Here's how the part is built. I have some questions about the finished solid (model axes, mm). Round coordinates to 2 decimals unless told otherwise and drop trailing zeros. Write each loop counter-clockwise with the first axis right and the second up, starting at its lowest first coordinate (ties: lowest second). Pieces come first, ordered by that corner, then holes. Notation, with made-up numbers: (-13, -12) -> (19, -12) arc R23 ccw to (19, 17) -> close; hole circle Ø2 at (-15.75, 36). An arc over 180 degrees is marked (long way). Answer in a Markdown table with one row per item.
from build123d import *

# Parameters (mm, degrees)
F0_R     = 15.875
F1_DEPTH = 25.4


with BuildPart() as f1:
    # F0 (on Front) → F1 (new body)
    with BuildSketch(Plane.XZ):
        with BuildLine():
            ThreePointArc((-49.0055754781, -12.3038528651), (-41.5660877202, -30.2643651072), (-23.6055754781, -37.7038528651))
            Line((-23.6055754781, -37.7038528651), (-23.3435511934, -37.7038528651))
            Line((-23.3435511934, -37.7038528651), (42.6555754781, -37.7038528651))
            ThreePointArc((42.6555754781, -37.7038528651), (60.6160877202, -30.2643651072), (68.0555754781, -12.3038528651))
            ThreePointArc((68.0555754781, -12.3038528651), (66.5394936483, -3.6598692442), (62.1722327349, 3.9522256755))
            Line((62.1722327349, 3.9522256755), (31.7932017285, 51.9582280247))
            Line((31.7932017285, 51.9582280247), (30.1001638771, 54.6336253754))
            ThreePointArc((30.1001638771, 54.6336253754), (9.0757549966, 65.1359410719), (-11.5640531978, 53.8966029481))
            Line((-11.5640531978, 53.8966029481), (-12.2938214906, 52.7437224792))
            Line((-12.2938214906, 52.7437224792), (-43.3631999383, 3.6606368673))
            ThreePointArc((-43.3631999383, 3.6606368673), (-47.5104832797, -3.714089206), (-49.0055754781, -12.0418285804))
            Line((-49.0055754781, -12.0418285804), (-49.0055754781, -12.3038528651))
        make_face()
        with Locations((-23.6055754781, -12.3038528651)):
            Circle(F0_R, mode=Mode.SUBTRACT)
        with BuildLine():
            ThreePointArc((26.7805754781, -12.3038528651), (42.6555754781, 3.5711471349), (58.5305754781, -12.3038528651))
            ThreePointArc((58.5305754781, -12.3038528651), (42.6555754781, -28.1788528651), (26.7805754781, -12.3038528651))
        make_face(mode=Mode.SUBTRACT)
        with Locations((9.525, 39.7399142385)):
            Circle(F0_R, mode=Mode.SUBTRACT)
        with BuildLine():
            Line((-23.3435511934, -37.7038528651), (-23.6055754781, -37.7038528651))
            ThreePointArc((-23.6055754781, -37.7038528651), (-41.5660877202, -30.2643651072), (-49.0055754781, -12.3038528651))
            Line((-49.0055754781, -12.3038528651), (-49.0055754781, -12.0418285804))
            ThreePointArc((-49.0055754781, -12.0418285804), (-41.5670433569, -30.2653207439), (-23.3435511934, -37.7038528651))
        make_face()
        with BuildLine():
            ThreePointArc((-11.5640531978, 53.8966029481), (-11.936680058, 53.3250638176), (-12.2938214906, 52.7437224792))
            Line((-12.2938214906, 52.7437224792), (-11.5640531978, 53.8966029481))
        make_face()
        with BuildLine():
            Line((30.1001638771, 54.6336253754), (31.7932017285, 51.9582280247))
            ThreePointArc((31.7932017285, 51.9582280247), (30.9884091386, 53.3223318491), (30.1001638771, 54.6336253754))
        make_face()
    extrude(amount=F1_DEPTH)


solid = f1.part
1) I want a section at B-B, the plane x = 15. List the corners of the cut face in (y, z) for me.
Response:
| item | result |
|---|---|
| outline | (-25.4, -37.7) -> (0, -37.7) -> (0, 24.84) -> (-25.4, 24.84) -> close; (-25.4, 54.64) -> (0, 54.64) -> (0, 64.54) -> (-25.4, 64.54) -> close |
2) I want a section at A-A, the plane z = 48. List the corners of the cut face in (x, y) for me, and give its area (3 significant figures).
Response:
| item | result |
|---|---|
| outline | (-15.3, -25.4) -> (-4.03, -25.4) -> (-4.03, 0) -> (-15.3, 0) -> close; (23.08, -25.4) -> (34.3, -25.4) -> (34.3, 0) -> (23.08, 0) -> close |
| area | 571 mm^2 |
3) I want a section at C-C, the plane z = 1.5. List the corners of the cut face in (x, y) for me.
Response:
| item | result |
|---|---|
| outline | (-44.93, -25.4) -> (-31.45, -25.4) -> (-31.45, 0) -> (-44.93, 0) -> close; (-15.77, -25.4) -> (34.82, -25.4) -> (34.82, 0) -> (-15.77, 0) -> close; (50.5, -25.4) -> (63.98, -25.4) -> (63.98, 0) -> (50.5, 0) -> close |
4) I want a section at D-D, the plane y = -6. List the corners of the cut face in (x, z) for me (3 decimals), and give its area (3 significant figures).
Response:
| item | result |
|---|---|
| outline | (-43.363, 3.661) arc R25.401 ccw to (-23.344, -37.704) -> (42.656, -37.704) arc R25.4 ccw to (62.172, 3.952) -> (31.793, 51.958) arc R25.4 ccw to (-12.294, 52.744) -> close; hole circle Ø31.75 at (-23.606, -12.304); hole circle Ø31.75 at (9.525, 39.74); hole circle Ø31.75 at (42.656, -12.304) |
| area | 6,180 mm^2 |
5) For pin 1 (8 mm diameter, centred on y = -22.5, z = 49, fed in from +X); pin 2 (8 mm diameter, centred on y = -9.5, z = 39, fed in from +X); pin 3 (3 mm diameter, centred on y = -6.5, z = 30.5, fed in from +X), each with a flat end and sliding along its axis, tell me the tip position at first contact or that it passes through.
Response:
| item | result |
|---|---|
| pin 1 | stops at x = 36.2 |
| pin 2 | stops at x = 42.52 |
| pin 3 | stops at x = 46.32 |
6) We'd pull the mould along X, two halves only. Please class faces 1 (the face through (47.195, -12.522, 27.619)), 2 (the face through (9, -13, -37.704)), 3 (the face through (-8.94, -12.52, -18.38)): +X half, -X half, draft (parallel to the pull), parting line (faces both ways), or undercut.
Response:
| item | result |
|---|---|
| face 1 | +X half |
| face 2 | draft |
| face 3 | undercut |
7) I need wall thicknesses on line 1 (X direction, y = -2, z = -3); line 2 (X direction, y = -9.25, z = -5); line 3 (Z direction, x = 22, y = -20.5). Which ranges of each line are inside material? Lowest first, please. Write a range as [from, to].
Response:
| item | result |
|---|---|
| line 1 | x = [-47.24, -36.47], [-10.74, 29.79], [55.52, 66.29] |
| line 2 | x = [-47.93, -37.7], [-9.51, 28.56], [56.75, 66.98] |
| line 3 | z = [-37.7, 29.92], [49.56, 61.87] |
